Source: CAD feature listing. Evaluate the final solid. Frame: model axes, mm. Face numbers are marked on the shaded views. A direction names the side the tool comes from. Give positions to 0.01 mm unless a question says otherwise; leave off trailing zeros. Order: outer loops, then holes, each group sorted by start corner. A loop starts at its lowest first (then second) coordinate and runs counter-clockwise, first axis right, second up.
Autodesk Inventor part; units mm, degrees
ref_plane "YZ Plane" through (0, 0, 0) normal (1, 0, 0) x (0, 1, 0)
ref_plane "XZ Plane" through (0, 0, 0) normal (0, 1, 0) x (-1, 0, 0)
ref_plane "XY Plane" through (0, 0, 0) normal (0, 0, 1) x (1, 0, 0)
sketch "Esquisse1" plane through (0, 0, 0) normal (0, 0, 1) x (1, 0, 0)
  line L0 (-186.69, 0) -> (186.69, 0)
  line L1 (0, -197.485) -> (0, 251.46)
  circle A0 centre (0, 0) radius 133.35 construction
  line L2 (-50.292, 138.9194) -> (-50.292, 88.9302)
  line L3 (50.292, 88.9302) -> (50.292, 138.9194)
  line L4 (-5.4717, 146.4909) -> (0, 146.4909)
  line L5 (-59.3639, 174.3189) -> (62.2899, 174.3189) construction
  line L6 (62.2899, 174.3189) -> (62.2899, 74.4875) construction
  line L7 (62.2899, 74.4875) -> (-59.3639, 74.4875) construction
  line L8 (-59.3639, 74.4875) -> (-59.3639, 174.3189) construction
  line L9 (-46.6745, 139.3954) -> (-43.813, 136.0491)
  line L10 (-41.4, 134.9375) -> (-21.2184, 134.9375)
  line L11 (-14.2687, 139.0403) -> (-12.4215, 142.3881)
  line L12 (0, 14.2875) -> (0, 187.325) construction
  arc A1 (-46.6745, 139.3954) -> (-48.8631, 140.499) centre (-49.0875, 137.3319) ccw
  arc A2 (-43.813, 136.0491) -> (-41.4, 134.9375) centre (-41.4, 138.1125) ccw
  arc A3 (-48.8631, 140.499) -> (-50.292, 138.9194) centre (-48.7045, 138.9194) ccw
  arc A4 (-21.2184, 134.9375) -> (-14.2687, 139.0403) centre (-21.2184, 142.875) ccw
  arc A5 (-5.4717, 146.4909) -> (-12.4215, 142.3881) centre (-5.4717, 138.5534) ccw
  line L13 (5.4717, 146.4909) -> (0, 146.4909)
  line L14 (46.6745, 139.3954) -> (43.813, 136.0491)
  line L15 (41.4, 134.9375) -> (21.2184, 134.9375)
  line L16 (14.2687, 139.0403) -> (12.4215, 142.3881)
  arc A6 (48.8631, 140.499) -> (46.6745, 139.3954) centre (49.0875, 137.3319) ccw
  arc A7 (41.4, 134.9375) -> (43.813, 136.0491) centre (41.4, 138.1125) ccw
  arc A8 (50.292, 138.9194) -> (48.8631, 140.499) centre (48.7045, 138.9194) ccw
  arc A9 (14.2687, 139.0403) -> (21.2184, 134.9375) centre (21.2184, 142.875) ccw
  arc A10 (12.4215, 142.3881) -> (5.4717, 146.4909) centre (5.4717, 138.5534) ccw
  line L17 (-48.7045, 87.3427) -> (-25.6128, 87.3427)
  arc A11 (0, 90.4875) -> (-25.1966, 87.3982) centre (-1.8902, 1.6076) ccw
  arc A12 (-50.292, 88.9302) -> (-48.7045, 87.3427) centre (-48.7045, 88.9302) ccw
  arc A13 (-25.6128, 87.3427) -> (-25.1966, 87.3982) centre (-25.6128, 88.9302) ccw
  line L18 (48.7045, 87.3427) -> (25.6128, 87.3427)
  arc A14 (25.1966, 87.3982) -> (0, 90.4875) centre (1.8902, 1.6076) ccw
  arc A15 (25.1966, 87.3982) -> (25.6128, 87.3427) centre (25.6128, 88.9302) ccw
  arc A16 (48.7045, 87.3427) -> (50.292, 88.9302) centre (48.7045, 88.9302) ccw
  point P0 (-25.4, 87.3427)
  point P1 (48.7045, 87.3427)
  dimension "d0" = 266.7
  dimension "d1" = 100.584
  dimension "d37" = 121.6538
  dimension "d38" = 99.8314
  dimension "d39" = 74.4875
  dimension "d40" = 59.3639
  dimension "d52" = 3.175
  dimension "d55" = 1.5875
  dimension "d58" = 7.9375
  dimension "d67" = 88.9
  dimension "d68" = 1.5875
  dimension "d72" = 1.5875
extrude "Extrusion1" add sketch "Esquisse1" along normal blind 3.175
sketch "Esquisse2" plane through (0, 0, 0) normal (0, 0, -1) x (-1, 0, 0)
  line L0 (-50.292, 138.9194) -> (-50.292, 88.9302)
  line L1 (-21.2184, 134.9375) -> (-41.4, 134.9375)
  line L2 (-48.2586, 90.2748) -> (-48.2586, 122.0318)
  line L3 (-46.6734, 88.6873) -> (-26.9271, 88.6585)
  arc A0 (0, 91.9607) -> (-26.9271, 88.6585) centre (1.948, -35.3617) ccw
  arc A1 (0, 133.35) -> (-46.2034, 125.0028) centre (-0.3874, 3.4484) ccw
  line L4 (0, -197.485) -> (0, 251.46)
  line L5 (48.2586, 90.2748) -> (48.2586, 122.0318)
  line L6 (46.6734, 88.6873) -> (27.1101, 88.6588)
  arc A2 (26.75, 88.6996) -> (0, 91.9607) centre (-1.948, -35.3617) ccw
  arc A3 (46.2034, 125.0028) -> (0, 133.35) centre (0.3874, 3.4484) ccw
  arc A4 (-48.2586, 90.2748) -> (-46.6734, 88.6873) centre (-46.6711, 90.2748) ccw
  arc A5 (26.75, 88.6996) -> (27.1101, 88.6588) centre (27.1078, 90.2463) ccw
  arc A6 (46.6734, 88.6873) -> (48.2586, 90.2748) centre (46.6711, 90.2748) ccw
  arc A7 (-46.2034, 125.0028) -> (-48.2586, 122.0318) centre (-45.0836, 122.0318) ccw
  arc A8 (48.2586, 122.0318) -> (46.2034, 125.0028) centre (45.0836, 122.0318) ccw
  point P0 (0, 0)
  point P1 (-48.2586, 88.6897)
  point P2 (-48.2586, 124.2082)
  point P3 (48.2586, 88.6897)
  point P4 (48.2586, 124.2082)
  point P5 (26.9271, 88.6585)
  dimension "d80" = 1.5875
  dimension "d81" = 3.175
extrude "Extrusion2" add sketch "Esquisse2" along normal blind 9.271
sketch "Esquisse3" plane through (0, 0, 0) normal (0, 0, -1) x (-1, 0, 0)
  circle A0 centre (0, 141.7847) radius 2.1822
  point P0 (0, 0)
extrude "Extrusion3" cut sketch "Esquisse3" against normal blind 9.271
equation "\"d0\" = para_d"
equation "\"para_a\" = 25.4"
equation "\"para_b\" = 25.4"
equation "\"para_c\" = 25.4"
equation "\"para_d\" = 266.7"
equation "\"para_e\" = 25.4"
properties part number "BRAKE PAD" material "Acier"
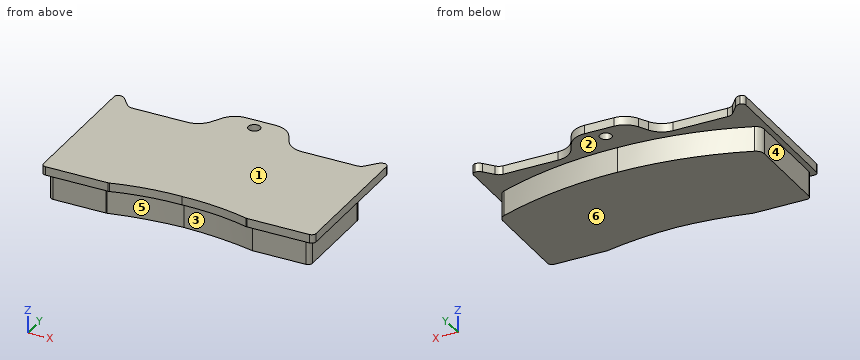
1) Pin query (flat end, axial travel): pin 1 (1 mm diameter, centred on x = -22, z = -1.5, fed in from -Y); pin 2 (1 mm diameter, centred on x = 33, z = 2, fed in from +Y); pin 3 (3.5 mm diameter, centred on x = 0, y = 141.78, fed in from -Z) (3 decimals); pin 4 (2 mm diameter, centred on x = 6, z = 0.5, fed in from -Y). Return the tip coordinate at first contact, or that it passes through.
Report:
pin 1: stops at y = 89.61
pin 2: stops at y = 134.94
pin 3: passes through
pin 4: stops at y = 90.36
2) Reachability of the marked faces 1 and 2 from +Z, -Z, +X, -X, +Y, -Y: full face, straight path, thin tool, end or side. Return the list, or none.
Report:
face 1: +Z, +X, -X, +Y, -Y
face 2: -Z
3) Material intervals for L1, parallel to Y at x = 0, z = 1.2; L2, parallel to X at y = 106.5, z = -0.5; L3, parallel to Z at x = -18, y = 135.5 (3 decimals), sorted ascending.
Report:
L1: y = 90.49 to 139.6, 143.97 to 146.49
L2: x = -48.26 to 48.26
L3: z = 0 to 3.175
4) Section query A-A, the plane y = 105.5. Return the cut outline in (x, z) (3 decimals).
Report:
outline: (-50.292, 0) - (-48.259, 0) - (-48.259, -9.271) - (48.259, -9.271) - (48.259, 0) - (50.292, 0) - (50.292, 3.175) - (-50.292, 3.175) - close
5) Draft query along X for the marked faces 3, 4, 5 and 6. Return one class per face: +X half, -X half, draft (parallel to the pull), parting line (faces both ways), or undercut.
Report:
face 3: undercut
face 4: -X half
face 5: undercut
face 6: draft
6) Section query C-C, the plane x = 39.5. Return the cut outline in (y, z) (1 decimal).
Report:
outline: (87.3, 0) - (88.7, 0) - (88.7, -9.3) - (127.3, -9.3) - (127.3, 0) - (134.9, 0) - (134.9, 3.2) - (87.3, 3.2) - close
